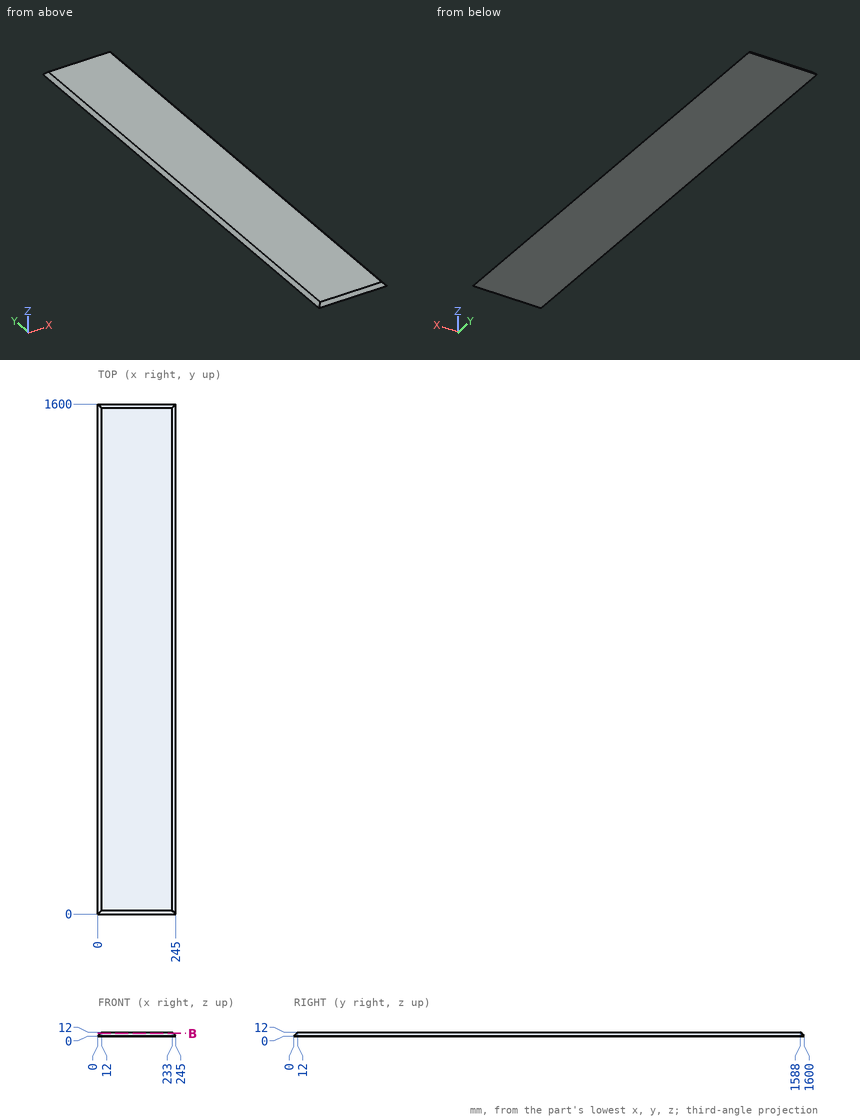
Answer from the drawing. Dimensions are ordinates in mm from the lowest x, y and z of the part. Give positions to 0.01 mm unless a question says otherwise; leave off trailing zeros. Order: outer loops, then holes, each group sorted by start corner. A loop starts at its lowest first (then second) coordinate and runs counter-clockwise, first axis right, second up.
(1) Straight lines are drawn through the part: L1, parallel to Y at x = 73, z = 11.75; L2, parallel to Y at x = 225, z = 1.5; L3, parallel to X at y = 1187.5, z = 4.25. For each, find the intervals that lie inside material, in ascending order.
(2) Given pin 1 (4 mm diameter, centred on y = 418.5, z = 6, fed in from +X); pin 2 (1 mm diameter, centred on y = 629.5, z = 9, fed in from -X), each flat-ended and moving along its own axis, determine where each tip first touches the part or whether it passes through.
(3) Find section B-B (z = 8.25). Give the vertices of the cut face in (x, y).
Result sheet:
1. L1: y = 11.75 to 1588.25
1. L2: y = 1.5 to 1598.5
1. L3: x = 4.25 to 240.75
2. pin 1: stops at x = 241
2. pin 2: stops at x = 8.5
3. outline: (8.25, 8.25) - (236.75, 8.25) - (236.75, 1591.75) - (8.25, 1591.75) - close
